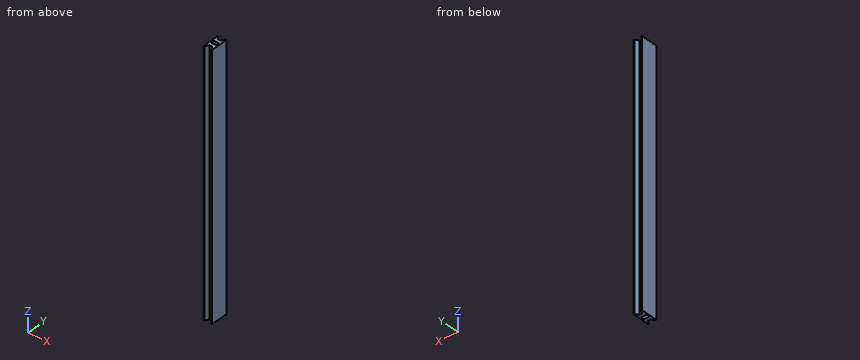
Autodesk Inventor part; units mm, degrees
ref_plane "YZ Plane" through (0, 0, 0) normal (1, 0, 0) x (0, 1, 0)
ref_plane "XZ Plane" through (0, 0, 0) normal (0, 1, 0) x (-1, 0, 0)
ref_plane "XY Plane" through (0, 0, 0) normal (0, 0, 1) x (1, 0, 0)
sketch "Sketch1" plane through (0, 0, 0) normal (0, 0, 1) x (1, 0, 0)
  line L0 (0, 0) -> (50, 0)
  line L1 (50, 0) -> (50, 100)
  line L2 (50, 100) -> (0, 100)
  line L3 (0, 100) -> (0, 0)
  dimension "d0" = 50
  dimension "d1" = 100
extrude "Extrusion1" add sketch "Sketch1" along normal blind 1500
sketch "Sketch2" plane through (0, 0, 1500) normal (0, 0, 1) x (1, 0, 0)
  line L0 (0, 0) -> (50, 0)
  line L1 (50, 0) -> (50, 100)
  line L2 (50, 100) -> (0, 100)
  line L3 (0, 100) -> (0, 0)
  line L4 (16.6667, 80) -> (33.3333, 80)
  line L5 (16.6667, 80) -> (43.3333, 80) construction
  line L6 (16.6667, 80) -> (5.1197, 100)
  line L7 (50, 100) -> (0, 100)
  line L8 (16.6667, 80) -> (39.7607, 80) construction
  line L9 (33.3333, 80) -> (44.8803, 100)
  line L10 (33.3333, 80) -> (56.4273, 80) construction
  line L11 (44.8803, 100) -> (5.1197, 100)
  line L12 (0, 50) -> (50, 50)
  line L13 (50, 0) -> (50, 100)
  line L14 (16.6667, 20) -> (33.3333, 20)
  line L15 (16.6667, 20) -> (5.1197, 0)
  line L16 (33.3333, 20) -> (44.8803, 0)
  line L17 (44.8803, 0) -> (5.1197, 0)
  dimension "d4" = 50
  dimension "d5" = 16.6667
  dimension "d6" = 100
  dimension "d7" = 20
  dimension "d8" = 16.6667
  dimension "d11" = 120
  dimension "d12" = 60
  dimension "d13" = 50
extrude "Extrusion2" cut sketch "Sketch2" against normal up to next contours L15 L14 L16 L0 | L2 L9 L4 L6
sketch "Sketch3" plane through (0, 0, 1500) normal (0, 0, 1) x (1, 0, 0)
  line L0 (33.3333, 80) -> (16.6667, 80)
  line L1 (16.6667, 60) -> (33.3333, 60)
  line L2 (0, 100) -> (0, 0)
  line L3 (16.6667, 20) -> (33.3333, 20)
  line L4 (50, 100) -> (44.8803, 100)
  line L5 (16.6667, 40) -> (33.3333, 40)
  line L6 (5.1197, 56.6667) -> (5.1197, 43.3333)
  line L7 (25, 80) -> (25, 20)
  line L8 (16.6667, 60) -> (5.1197, 56.6667)
  line L9 (16.6667, 40) -> (5.1197, 43.3333)
  line L10 (44.8803, 56.6667) -> (44.8803, 43.3333)
  line L11 (33.3333, 60) -> (44.8803, 56.6667)
  line L12 (33.3333, 40) -> (44.8803, 43.3333)
  dimension "d16" = 16.6667
  dimension "d17" = 16.6667
  dimension "d18" = 16.6667
  dimension "d19" = 16.6667
  dimension "d20" = 20
  dimension "d21" = 20
  dimension "d22" = 100
  dimension "d23" = 16.6667
  dimension "d25" = 40
  dimension "d26" = 16.6667
  dimension "d27" = 13.3333
  dimension "d28" = 3.3333
extrude "Extrusion3" cut sketch "Sketch3" against normal blind 2900
equation "\"d1\" = 2 * d0"
equation "\"d5\" = 0.333333 * d4"
equation "\"d7\" = 0.2 * d6"
equation "\"d8\" = -0.5 * d5 + 0.5 * d4"
equation "\"d13\" = 0.5 * d6"
equation "\"d17\" = d16"
equation "\"d19\" = d18"
equation "\"d21\" = 0.5 * d22 - 1.5 * d20"
equation "\"d23\" = d24"
equation "\"d25\" = -0.5 * d20 + 0.5 * d22"
equation "\"d26\" = d16"
equation "\"d27\" = 0.666667 * d21"
equation "\"d28\" = -0.5 * d27 + 0.5 * d21"
properties part number "wheelRoadGantry"
The listing builds one solid part. Answer for the finished solid, in the listing's coordinates (mm). Give positions to 0.01 mm unless a question says otherwise; leave off trailing zeros. Write each loop counter-clockwise with the first axis right and the second up, starting at its lowest first coordinate (ties: lowest second). Pieces come first, ordered by that corner, then holes. Notation, with made-up numbers: M 27.25,-34.75 L 38.25,-34.75 A24 ccw 38.25,-5.75 Z; hole C 39.25,87.25 d11. An arc over 180 degrees is marked long. Write each question's results on one line, items separated by ' | '.
Q1. Section A-A, the plane z = 290 is taken. Write down the section's boundary in (x, y).
Output values:
outline: M 0,0 L 5.12,0 L 16.67,20 L 33.33,20 L 44.88,0 L 50,0 L 50,100 L 44.88,100 L 33.33,80 L 16.67,80 L 5.12,100 L 0,100 Z; hole M 5.12,43.33 L 16.67,40 L 33.33,40 L 44.88,43.33 L 44.88,56.67 L 33.33,60 L 16.67,60 L 5.12,56.67 Z
Q2. Consider L1, parallel to X at y = 56.5, z = 699; L2, parallel to Y at x = 24, z = 1323.5; L3, parallel to X at y = 19.5, z = 67. Determine where each line is inside the solid, lowest interval first. Write a range as from..to.
Output values:
L1: 0..5.12, 44.88..50 | L2: 20..40, 60..80 | L3: 0..16.38, 33.62..50
Q3. Flat-ended cylindrical pins translate along their axes: P1, Ø6, axis at x = 24.5, z = 296.5, coming from the +Y side; P2, Ø13.5, axis at x = 23, z = 566, coming from the +Y side; P3, Ø5, axis at x = 35.5, z = 431, coming from the +Y side. Find the tip coordinate at first contact, or state that the pin passes through.
Output values:
P1: y = 80 | P2: y = 80.72 | P3: y = 88.08
